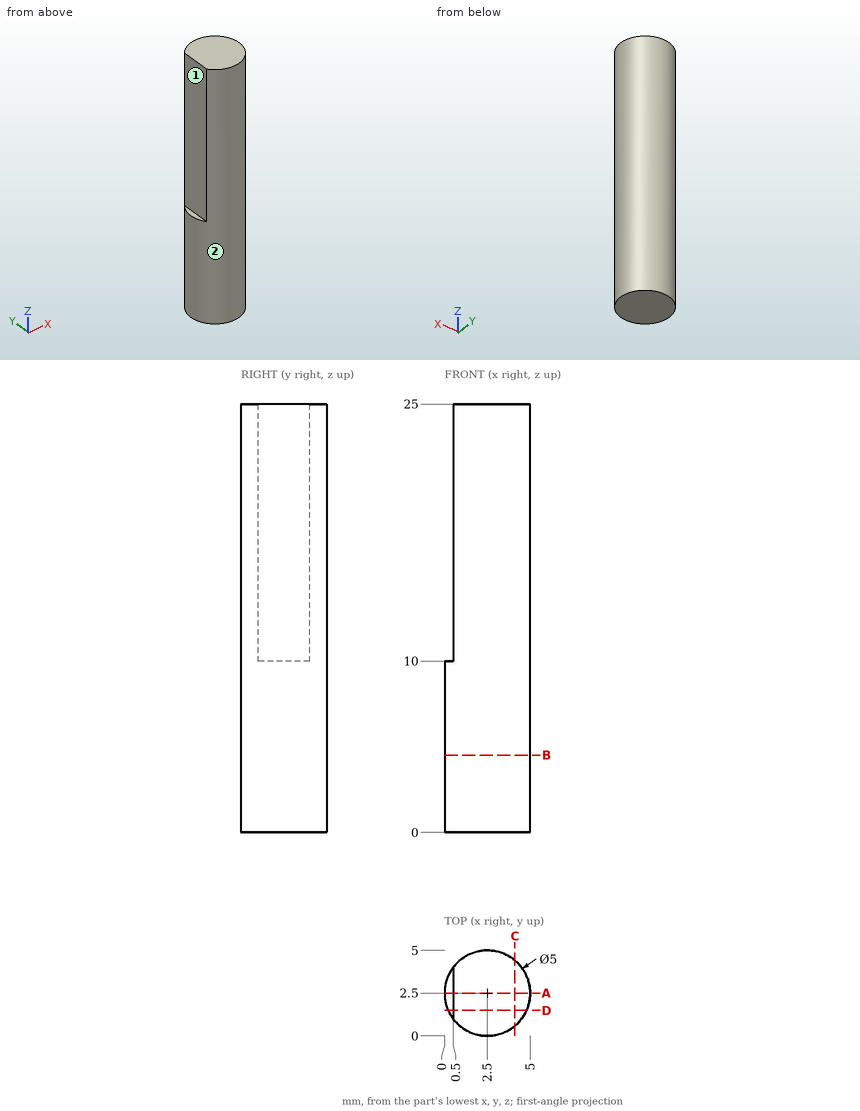
Design review of the part shown in the three views and the two pictorial views. Dimensions are in mm from the part's minimum x, y and z. A direction names the side the tool comes from. Round coordinates to 2 decimals unless told otherwise and drop trailing zeros. Order: outer loops, then holes, each group sorted by start corner. A loop starts at its lowest first (then second) coordinate and runs counter-clockwise, first axis right, second up. Notation, with made-up numbers: (-29, 20) -> (0, 20) arc R20 cw to (0, 32) -> close; hole circle Ø10 at (8.5, 78.5). An arc over 180 degrees is marked (long way). Write item = value, one per line. Start each with the question number.
1) Insertion check: pin 1 (3 mm diameter, centred on y = 1.5, z = 13.5, fed in from -X); pin 2 (0.6 mm diameter, centred on x = 0, y = 2.5, fed in from +Z). Each pin has a flat end and moves straight along its axis. Give the tip position at first contact, or say it passes through.
2) To check wall thickness, follow line 1 (X direction, y = 2.85, z = 21.5); line 2 (Y direction, x = 3.55, z = 3); line 3 (X direction, y = 4.3, z = 14.5). State the ranges of each line that lie inside material, in increasing order. Write a range as from..to.
3) Take a section at C-C on x = 4.1. State the section outline as (y, z) points, plus the area to 3 significant figures.
4) Take a section at A-A on y = 2.5. State the section outline as (x, z) points.
5) Tool access review of the marked faces 1 and 2: name each direction out of +Z, -Z, +X, -X, +Y, -Y from which nothing blocks a thin tool from reaching the whole face with its end or side.
6) Take a section at B-B on z = 4.5. State the section outline as (x, y) points.
7) Take a section at D-D on y = 1.5. State the section outline as (x, z) points.
Verdict:
q1.pin_1 = 0.5
q1.pin_2 = 10
q2.line_1 = 0.5..4.98
q2.line_2 = 0.23..4.77
q2.line_3 = 0.77..4.23
q3.outline = (0.58, 0) -> (4.42, 0) -> (4.42, 25) -> (0.58, 25) -> close
q3.area = 96.0 mm2
q4.outline = (0, 0) -> (5, 0) -> (5, 25) -> (0.5, 25) -> (0.5, 10) -> (0, 10) -> close
q5.face_1 = +Z, -X, +Y, -Y
q5.face_2 = +Z, -Z
q6.outline = circle Ø5 at (2.5, 2.5)
q7.outline = (0.21, 0) -> (4.79, 0) -> (4.79, 25) -> (0.5, 25) -> (0.5, 10) -> (0.21, 10) -> close
